CAD build for the part. Positions are in the model's coordinates, mm. Face numbers are marked on the shaded views. Round coordinates to 2 decimals unless told otherwise and drop trailing zeros. Write each loop counter-clockwise with the first axis right and the second up, starting at its lowest first coordinate (ties: lowest second). Pieces come first, ordered by that corner, then holes. Notation, with made-up numbers: (-39.75, 86.5) - (-12.75, 86.5) arc R28 ccw to (-12.75, 117.5) - close; hole circle Ø4 at (63.5, -14). An arc over 180 degrees is marked (long way). Answer in a Markdown table with one row per item.
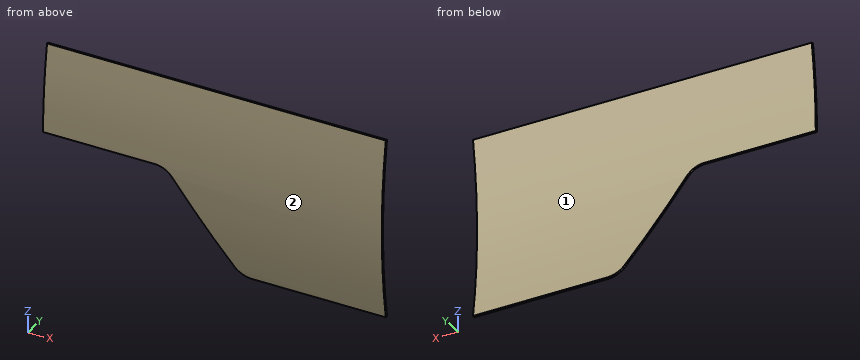
Autodesk Inventor part; units mm, degrees
ref_plane "YZ Plane" through (0, 0, 0) normal (1, 0, 0) x (0, 1, 0)
ref_plane "XZ Plane" through (0, 0, 0) normal (0, 1, 0) x (-1, 0, 0)
ref_plane "XY Plane" through (0, 0, 0) normal (0, 0, 1) x (1, 0, 0)
sketch "スケッチ1" plane through (0, 0, 0) normal (1, 0, 0) x (0, 1, 0)
  arc A0 (7.0384, 125) -> (7.0384, -125) centre (780.277, 0) ccw
  arc A1 (10, 124.5212) -> (10, -124.5212) centre (780.277, 0) ccw
  line L0 (10, 124.5212) -> (7.0384, 125)
  line L1 (10, -124.5212) -> (7.0384, -125)
  line L2 (0, -175) -> (0, 175)
  line L3 (10, 124.5212) -> (10, -124.5212)
  point P0 (0, 0)
  point P1 (0, 0)
  dimension "d0" = 3
  dimension "d1" = 250
  dimension "d2" = 10
extrude "押し出し1" add sketch "スケッチ1" along normal mid plane 470 contours L0 A1 L2 A0 | L2 A0 | L2 A1 L1 A0
sketch "スケッチ2" plane through (0, 0, 0) normal (0, 1, 0) x (-1, 0, 0)
  line L0 (65, 5) -> (235, 5)
  line L1 (235, -125) -> (-235, -125)
  line L2 (235, 124.5212) -> (235, -124.5212)
  line L3 (235, -124.5212) -> (-235, -124.5212)
  line L4 (-235, 125) -> (235, 125)
  line L5 (65, 5) -> (-35, -125)
  line L6 (-235, -124.5212) -> (-235, 124.5212)
  line L7 (235, 5) -> (235, -125)
  line L8 (-35, -125) -> (235, -125)
  point P0 (0, 0)
  dimension "d5" = 120
  dimension "d6" = 200
  dimension "d7" = 300
extrude "押し出し2" cut sketch "スケッチ2" along normal through all both and the other way through all
fillet "フィレット1" radius 30 2 edges at (-65, -1.484, 5) (34.8159, 8.5192, -124.7606)
properties part number "type7_element_base" material "CFRP"
Q1. Drill centre lines: line 1 (Y direction, x = 4, z = -7); line 2 (X direction, y = 1, z = -74); line 3 (Y direction, x = 64, z = -99). Where is each one in solid material? Low to high.
Computed:
| item | result |
|---|---|
| line 1 | y = -2.97 to 0.03 |
| line 2 | x = -4.23 to 235 |
| line 3 | y = 3.28 to 6.31 |
Q2. Saw through at C-C on z = 22. List the corners of the cut face in (x, y), then the cut area to 3 significant figures.
Computed:
| item | result |
|---|---|
| outline | (-235, -2.69) - (235, -2.69) - (235, 0.31) - (-235, 0.31) - close |
| area | 1,410 mm2 |
Q3. Pull direction Z, two halves, no side cores. Call the marked faces 1 and 2: released by +Z, released by -Z, zero draft, split by the parting line, or undercut.
Computed:
| item | result |
|---|---|
| face 1 | undercut |
| face 2 | split by the parting line |
Q4. Flat gauge pins, fed straight in: pin 1 (5 mm diameter, centred on x = -90, z = 53, fed in from -Y); pin 2 (0.9 mm diameter, centred on x = -153, y = -1, fed in from -Z). Where does each tip first touch, or does it go through?
Computed:
| item | result |
|---|---|
| pin 1 | stops at y = -1.37 |
| pin 2 | stops at z = 5 |
Q5. Saw through at B-B on x = 99. List the corners of the cut face in (y, z).
Computed:
| item | result |
|---|---|
| outline | (7.04, -125) - (10, -124.52) arc R780.28 cw to (10, 124.52) - (7.04, 125) arc R783.28 ccw to start |
